Here's how the part is built. I have some questions about the finished solid (model axes, mm). Give positions to 0.01 mm unless a question says otherwise; leave off trailing zeros. Loops run counter-clockwise (first coordinate to the right, second up) from the corner with the lowest first, then second, coordinate; pieces in that order, holes last.
Q1. Suppose I cut it at C-C (y = 2.3). List the corners of the cut face in (x, z) for me.
Q2. I need wall thicknesses on probe 1 along Z at (x, y) = (65, 2.5); probe 2 along X at (y, z) = (0.25, -110). Which ranges of each line are inside material? Lowest first, please.
Q3. Suppose I cut it at B-B (x = -58). List the corners of the cut face in (y, z) for me.
Q4. Suppose I cut it at A-A (z = -76). List the corners of the cut face in (x, y) for me.
Autodesk Inventor part; units mm, degrees
ref_plane "YZ Plane" through (0, 0, 0) normal (1, 0, 0) x (0, 1, 0)
ref_plane "XZ Plane" through (0, 0, 0) normal (0, 1, 0) x (-1, 0, 0)
ref_plane "XY Plane" through (0, 0, 0) normal (0, 0, 1) x (1, 0, 0)
sketch "Szkic1" plane through (0, 0, 0) normal (0, 1, 0) x (-1, 0, 0)
  line L0 (-169, -131.5) -> (169, -131.5)
  line L1 (169, -131.5) -> (169, 131.5)
  line L2 (169, 131.5) -> (-169, 131.5)
  line L3 (-169, 131.5) -> (-169, -131.5)
  line L4 (-169, -131.5) -> (169, 131.5) construction
  line L5 (169, -131.5) -> (-169, 131.5) construction
  point P0 (0, 0)
  dimension "d0" = 338
  dimension "d1" = 263
extrude "Wyciągnięcie proste1" add sketch "Szkic1" along normal blind 5
sketch "Szkic2" plane through (0, 0, 0) normal (0, -1, 0) x (1, 0, 0)
  line L0 (154, -116) -> (-154, -116)
  line L1 (-154, -116) -> (-154, 116)
  line L2 (-154, 116) -> (154, 116)
  line L3 (154, 116) -> (154, -116)
  line L4 (154, -116) -> (-154, 116) construction
  line L5 (-154, -116) -> (154, 116) construction
  point P0 (0, 0)
  dimension "d4" = 308
  dimension "d5" = 232
extrude "Wyciągnięcie proste2" cut sketch "Szkic2" against normal blind 10
fillet "Zaokrąglenie1" radius 2 4 edges at (-154, 2.5, 116) (-154, 2.5, -116) (154, 2.5, 116) (154, 2.5, -116)
fillet "Zaokrąglenie2" radius 5 4 edges at (169, 2.5, -131.5) (-169, 2.5, -131.5) (169, 2.5, 131.5) (-169, 2.5, 131.5)
properties part number "frame_upper" material "Tworzywo sztuczne PMMA"
Solutions:
1. outline: (-169, -126.5) arc R5 ccw to (-164, -131.5) - (164, -131.5) arc R5 ccw to (169, -126.5) - (169, 126.5) arc R5 ccw to (164, 131.5) - (-164, 131.5) arc R5 ccw to (-169, 126.5) - close; hole (-154, -114) arc R2 ccw to (-152, -116) - (152, -116) arc R2 ccw to (154, -114) - (154, 114) arc R2 ccw to (152, 116) - (-152, 116) arc R2 ccw to (-154, 114) - close
2. probe 1: z = -131.5 to -116, 116 to 131.5
2. probe 2: x = -169 to -154, 154 to 169
3. outline: (0, -131.5) - (5, -131.5) - (5, -116) - (0, -116) - close; (0, 116) - (5, 116) - (5, 131.5) - (0, 131.5) - close
4. outline: (-169, 0) - (-154, 0) - (-154, 5) - (-169, 5) - close; (154, 0) - (169, 0) - (169, 5) - (154, 5) - close
